Autodesk Inventor part; units mm, degrees
ref_plane "YZ Plane" through (0, 0, 0) normal (1, 0, 0) x (0, 1, 0)
ref_plane "XZ Plane" through (0, 0, 0) normal (0, 1, 0) x (-1, 0, 0)
ref_plane "XY Plane" through (0, 0, 0) normal (0, 0, 1) x (1, 0, 0)
sketch "草图1" plane through (0, 0, 0) normal (0, 0, 1) x (1, 0, 0)
  line L0 (0, 0) -> (14, 0)
  line L1 (14, 0) -> (14, -8)
  line L2 (14, -8) -> (0, -8)
  line L3 (0, -8) -> (0, 0)
  arc A0 (14, -8) -> (14, 0) centre (14, -4) ccw
  arc A1 (0, 0) -> (0, -8) centre (0, -4) ccw
  dimension "d0" = 14
  dimension "d1" = 8
extrude "拉伸1" add sketch "草图1" against normal blind 5
fillet "圆角1" radius 0.5 8 edges at (7, 0, 0) (-4, -4, 0) (7, -8, 0) (18, -4, 0) (7, -8, -5) (-4, -4, -5) (7, 0, -5) (18, -4, -5)
properties part number "装填盘轴键"
Geometry check sheet. Reference: the model listing, model coordinates, mm. Give positions to 0.01 mm unless a question says otherwise; leave off trailing zeros. Order: outer loops, then holes, each group sorted by start corner. A loop starts at its lowest first (then second) coordinate and runs counter-clockwise, first axis right, second up. Notation, with made-up numbers: (16, 25.5) - (53, 25.5) arc R33 cw to (53, 58.5) - close; hole circle Ø4 at (-3.5, 27). An arc over 180 degrees is marked (long way). Answer as a JSON object with one key per item and string values.
(1) Material ranges on line 1 (X direction, y = -4.5, z = -1); line 2 (Y direction, x = 16.5, z = -2.5); line 3 (X direction, y = -0.75, z = -0.65), recorded low to high.
Report:
{"line 1": "-3.97 to 17.97", "line 2": "-7.12 to -0.88", "line 3": "-2.33 to 16.33"}
(2) Cross-section at A-A (z = -2.75). Record the cut outline in (x, y).
Report:
{"outline": "(0, -8) - (14, -8) arc R4 ccw to (14, 0) - (0, 0) arc R4 ccw to start"}
(3) Depth check by flat-ended pin: pin 1 Ø1 at (y, z) = (-6.5, -1) entering from -X; pin 2 Ø2 at (y, z) = (-2.5, -4.5) entering from -X. Enter the tip coordinate at first touch or a pass-through.
Report:
{"pin 1": "x = -3.46", "pin 2": "x = -3.97"}
